Here's how the part is built. I have some questions about the finished solid (model axes, mm). Face numbers are marked on the shaded views. A direction names the side the tool comes from. Coordinates: 2 decimals unless noted, no trailing zeros. Write each loop counter-clockwise with the first axis right and the second up, starting at its lowest first coordinate (ties: lowest second). Pieces come first, ordered by that corner, then holes. Notation, with made-up numbers: (-39, -2.75) - (-12, -2.75) arc R18 ccw to (-12, 11.25) - close; hole circle Ø1 at (62.25, 21.5). An arc over 180 degrees is marked (long way). Answer in a Markdown table with one row per item. Add a question column.
Item 1: We'd pull the mould along Y, two halves only. Please class the marked faces 3, 4 and 5: +Y half, -Y half, draft (parallel to the pull), parting line (faces both ways), or undercut.
Item 2: Imagine slicing it at C-C (x = 0). Please give me the cut outline in (y, z).
Item 3: I'm going to push flat-ended pins straight in: pin 1 (1 mm diameter, centred on y = 5.5, z = -10.5, fed in from +X); pin 2 (2.5 mm diameter, centred on y = 6, z = -16, fed in from -X); pin 3 (3.5 mm diameter, centred on y = 6, z = -12.5, fed in from -X). Where does each tip first touch, or does it pass through?
Item 4: If I drill on probe 1 along X at (y, z) = (7, -18.5); probe 2 along X at (y, z) = (0, -7.75); probe 3 along Y at (x, z) = (1.4, -4), over which ranges is the centre line in solid material (lowest first)? Write a range as from..to.
Item 5: Which directions (+Z, -Z, +X, -X, +Y, -Y) give clear straight access to the entire face, cutting with the end or side of a thin tool? Please do the marked faces 1 and 2.
Item 6: Imagine slicing it at B-B (z = -16). State how many separate pieces and enclosed holes the cut face has, plus the area to 3 significant figures.
Item 7: Imagine slicing it at A-A (z = -9). Please give me the cut outline in (x, y), plus the area to 3 significant figures.
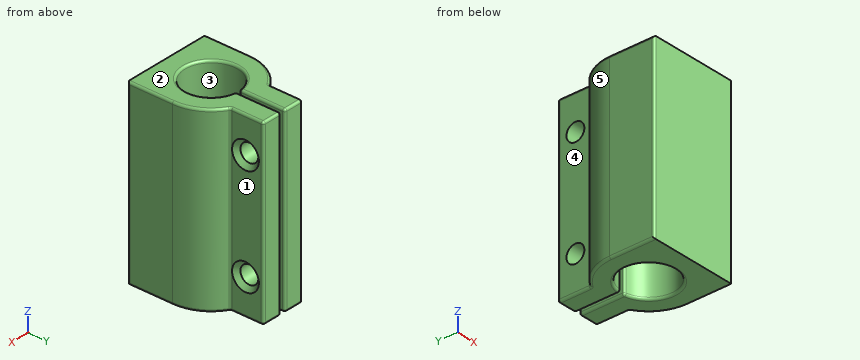
Autodesk Inventor part; units mm, degrees
ref_plane "YZ Plane" through (0, 0, 0) normal (1, 0, 0) x (0, 1, 0)
ref_plane "XZ Plane" through (0, 0, 0) normal (0, 1, 0) x (-1, 0, 0)
ref_plane "XY Plane" through (0, 0, 0) normal (0, 0, 1) x (1, 0, 0)
sketch "Sketch1" plane through (0, 0, 0) normal (0, 0, 1) x (1, 0, 0)
  arc A0 (-2.5, 4.3301) -> (2.5, 4.3301) centre (0, 0) ccw
  line L0 (2.5, 4.3301) -> (2.5, 8)
  line L1 (2.5, 8) -> (-2.5, 8)
  line L2 (-2.5, 8) -> (-2.5, 4.3301)
  circle A1 centre (0, 0) radius 2.95
  line L3 (-0.25, 8) -> (0.25, 8)
  line L4 (0.25, 8) -> (0.25, 2.5)
  line L5 (0.25, 2.5) -> (-0.25, 2.5)
  line L6 (-0.25, 2.5) -> (-0.25, 8)
  line L7 (-5, 0) -> (-5, -5)
  line L8 (-5, -5) -> (0, -5)
  line L9 (5, 0) -> (5, -5)
  line L10 (5, -5) -> (0, -5)
  point P0 (0.25, 2.9394)
  point P1 (-0.25, 2.9394)
  dimension "d0" = 10
  dimension "d1" = 5
  dimension "d2" = 2.5
  dimension "d3" = 8
  dimension "d4" = 3.6699
  dimension "d7" = 5.9
  dimension "d8" = 0.5
  dimension "d9" = 0.25
  dimension "d10" = 0
  dimension "d11" = 5.5
extrude "Extrusion1" add sketch "Sketch1" against normal blind 20 contours L2 L1 L6 A1 L4 L0 A0 | A0 L8 L7 | A0 L9 L10
sketch "Sketch2" plane through (2.5, 4.3301, 0) normal (1, 0, 0) x (0, 0, -1)
  circle A0 centre (4, 1.6699) radius 1
  circle A1 centre (16, 1.6699) radius 1
  line L0 (0, 0) -> (0, 3.6699)
  line L1 (20, 3.6699) -> (20, 0)
  line L2 (0, 3.6699) -> (20, 3.6699)
  point P0 (0, -4.3301)
  dimension "d12" = 2
  dimension "d13" = 4
  dimension "d14" = 2
  dimension "d15" = 4
  dimension "d16" = 2
  dimension "d17" = 2
extrude "Extrusion2" cut sketch "Sketch2" against normal up to surface (5 mm away)
chamfer "Chamfer1" distance 0.5 angle 45 2 edges at (2.5, 6, -3) (2.5, 6, -15)
fillet "Fillet1" radius 0.25 32 edges at (-0.25, 5.4697, 0) (0.25, 5.4697, 0) (-0.25, 8, -10) (0.25, 8, -10) (-1.375, 8, -20) (1.375, 8, -20) (-0.25, 5.4697, -20) (0.25, 5.4697, -20) (-1.375, 8, 0) (1.375, 8, 0) (-2.5, 8, -10) (-2.5, 6.1651, 0) (-2.5, 6.1651, -20) (2.5, 8, -10) (2.5, 6.1651, -20) (2.5, 6.1651, 0) (-5, -2.5, 0) (-4.3301, 2.5, 0) (5, -2.5, 0) (4.3301, 2.5, 0) (5, -2.5, -20) (4.3301, 2.5, -20) (0, -2.95, 0) (-5, -2.5, -20) (-4.3301, 2.5, -20) (0, -2.95, -20) (0.25, 2.9394, -10) (-0.25, 2.9394, -10) (-2.5, 4.3301, -10) (2.5, 4.3301, -10) (-5, -5, -10) (5, -5, -10)
properties part number "Holder"
Here are the results:
| question | item | result |
|---|---|---|
| 1 | face 3 | undercut |
| 1 | face 4 | draft |
| 1 | face 5 | +Y half |
| 2 | outline | (-5, -20) - (-3.2, -20) arc R0.25 ccw to (-2.95, -19.75) - (-2.95, -0.25) arc R0.25 ccw to (-3.2, 0) - (-5, 0) - close |
| 3 | pin 1 | stops at x = 2.5 |
| 3 | pin 2 | stops at x = -2.5 |
| 3 | pin 3 | stops at x = -2.63 |
| 4 | probe 1 | x = -2.5..-0.25, 0.25..2.5 |
| 4 | probe 2 | x = -5..-2.95, 2.95..5 |
| 4 | probe 3 | y = -5..-2.6, 2.6..5, 7..8 |
| 5 | face 1 | +Z, -Z, +X, +Y |
| 5 | face 2 | +Z, +X, -X, +Y, -Y |
| 6 | separate pieces | 3 |
| 6 | enclosed holes | 0 |
| 6 | area | 66.1 mm2 |
| 7 | outline | (-5, -4.75) arc R0.25 ccw to (-4.75, -5) - (4.75, -5) arc R0.25 ccw to (5, -4.75) - (5, 0) arc R5 ccw to (2.62, 4.26) arc R0.25 cw to (2.5, 4.47) - (2.5, 7.75) arc R0.25 ccw to (2.25, 8) - (0.5, 8) arc R0.25 ccw to (0.25, 7.75) - (0.25, 3.16) arc R0.25 ccw to (0.46, 2.91) arc R2.95 cw (long way) to (-0.46, 2.91) arc R0.25 ccw to (-0.25, 3.16) - (-0.25, 7.75) arc R0.25 ccw to (-0.5, 8) - (-2.25, 8) arc R0.25 ccw to (-2.5, 7.75) - (-2.5, 4.47) arc R0.25 cw to (-2.62, 4.26) arc R5 ccw to (-5, 0) - close |
| 7 | area | 75.4 mm2 |
